CAD build for the part. Positions are in the model's coordinates, mm. Give positions to 0.01 mm unless a question says otherwise; leave off trailing zeros. Loops run counter-clockwise (first coordinate to the right, second up) from the corner with the lowest first, then second, coordinate; pieces in that order, holes last. Notation, with made-up numbers: M -27,-19 L 3,-19 A20 cw 3,6 Z; hole C 41.25,3.25 d4. An arc over 180 degrees is marked long. One line per question, with ' | ' between items.
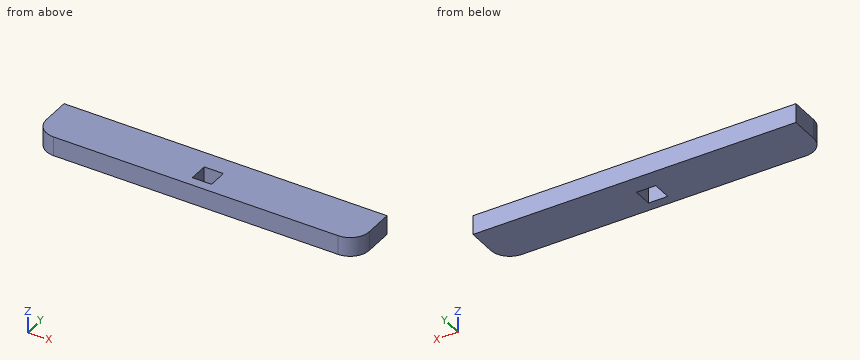
```python
from build123d import *

# Parameters (mm, degrees)
SKETCH1_W           = 3.175
SKETCH1_H           = 3.175
BOSS_EXTRUDE1_DEPTH = 3.175


with BuildPart() as part:
    # Sketch1 → Boss-Extrude1 (new body)
    with BuildSketch(Plane.XY):
        with BuildLine():
            Line((10.16, -2.286), (63.5, -2.286))
            Line((63.5, -2.286), (63.5, -6.985))
            ThreePointArc((63.5, -6.985), (62.57006403, -9.23006403), (60.325, -10.16))
            Line((60.325, -10.16), (13.335, -10.16))
            ThreePointArc((13.335, -10.16), (11.08993597, -9.23006403), (10.16, -6.985))
            Line((10.16, -6.985), (10.16, -2.286))
        make_face()
        with Locations((36.83, -6.985)):
            Rectangle(SKETCH1_W, SKETCH1_H, mode=Mode.SUBTRACT)
    extrude(amount=BOSS_EXTRUDE1_DEPTH)


solid = part.part
```
Item 1: Drill centre lines: line 1 along Y through (x, z) = (35.5, 0.7); line 2 along X through (y, z) = (-6.75, 0.5); line 3 along X through (y, z) = (-8.5, 1). Where is each one in solid material? Low to high. Write a range as [from, to].
Conclusion:
line 1: [-10.16, -8.57], [-5.4, -2.29] | line 2: [10.16, 35.24], [38.42, 63.5] | line 3: [10.54, 35.24], [38.42, 63.12]
Item 2: Saw through at C-C on y = -9.25. Give the cut face in (x, z) (3 decimals).
Conclusion:
outline: M 11.11,0 L 62.55,0 L 62.55,3.175 L 11.11,3.175 Z
Item 3: Saw through at A-A on y = -6. Give the cut face in (x, z) (1 decimal), and give its area (3 significant figures).
Conclusion:
outline: M 10.2,0 L 35.2,0 L 35.2,3.2 L 10.2,3.2 Z; M 38.4,0 L 63.5,0 L 63.5,3.2 L 38.4,3.2 Z | area: 159 mm²
